Print and shaded views of the part. All mm, measured from the part's lowest x, y and z. Round coordinates to 2 decimals unless told otherwise and drop trailing zeros. Order: outer loops, then holes, each group sorted by start corner. A loop starts at its lowest first (then second) coordinate and runs counter-clockwise, first axis right, second up. Notation, with made-up numbers: (5, 39.25) - (60, 39.25) arc R26 ccw to (60, 57.25) - close; hole circle Ø4 at (-19.5, -0.5). An arc over 180 degrees is marked (long way). Write item = value, one per line.
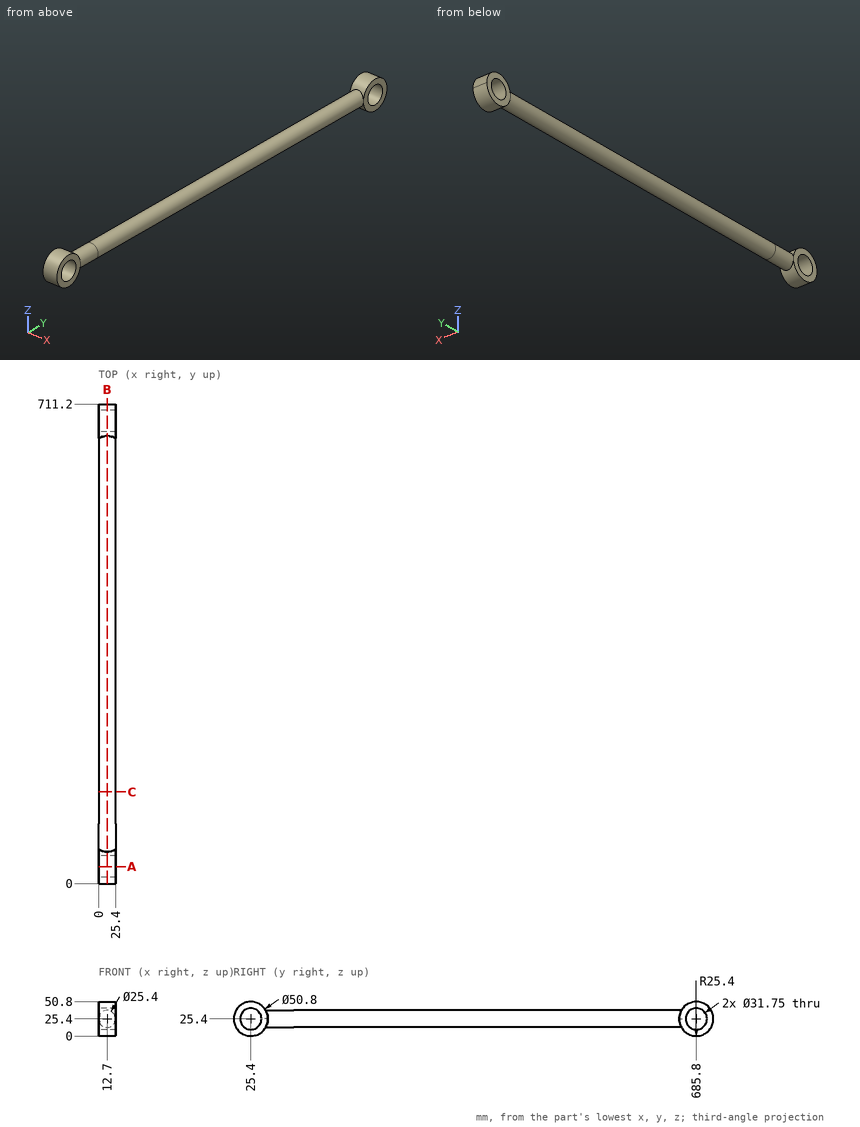
(1) Band-saw the part on C-C on y = 136. List the corners of the cut face in (x, z).
Solved:
outline = circle Ø25.4 at (12.7, 25.4)
(2) Band-saw the part on B-B on x = 12.7. List the corners of the cut face in (y, z) (3 decimals), plus the area to 3 significant figures.
Solved:
outline = (47.397, 12.7) - (663.803, 12.7) arc R25.4 ccw (long way) to (663.803, 38.1) - (47.397, 38.1) arc R25.4 ccw (long way) to start; hole circle Ø31.75 at (25.4, 25.4); hole circle Ø31.75 at (685.8, 25.4)
area = 18,000 mm²
(3) Band-saw the part on A-A on y = 25.4. List the corners of the cut face in (x, z) (3 decimals), plus the area to 3 significant figures.
Solved:
outline = (0, 0) - (25.4, 0) - (25.4, 9.525) - (0, 9.525) - close; (0, 41.275) - (25.4, 41.275) - (25.4, 50.8) - (0, 50.8) - close
area = 484 mm²
(4) Probe line 1 along Y through (x, z) = (18.75, 27); line 2 along Y through (x, z) = (2, 18); line 3 along Z through (x, y) = (15.25, 25.4) (3 decimals). List the from-to ranges inside material, lowest first.
Solved:
line_1 = 0.05 to 9.61, 41.19 to 670.01, 701.59 to 711.15
line_2 = 1.1 to 11.36, 39.44 to 49.7, 661.5 to 671.76, 699.84 to 710.1
line_3 = 0 to 9.525, 41.275 to 50.8
(5) Drop flat-ended pins along their axis: pin 1 (2 mm diameter, centred on y = 626.5, z = 23.5, fed in from -X); pin 2 (8 mm diameter, centred on x = 19.5, z = 11.5, fed in from -Y); pin 3 (5 mm diameter, centred on x = 18.5, y = 112, fed in from -Z). Give the stop position or say it passes through.
Solved:
pin_1 = 0.03
pin_2 = 2.01
pin_3 = 13.14
